```python
from build123d import *

# Parameters (mm, degrees)
BOSS_EXTRUDE1_DEPTH  = 6.5
SKETCH2_R            = 5.5
CUT_EXTRUDE2_DEPTH   = 5
SKETCH3_R            = 4
CUT_EXTRUDE4_DEPTH   = 1.5
M2_CLEARANCE_HOLE1_D = 2.4
M2_CLEARANCE_HOLE2_D = 2.4


with BuildPart() as part:
    # Sketch1 → Boss-Extrude1 (new body)
    with BuildSketch(Plane(origin=(0, 24.8, 0), x_dir=(1, 0, 0), z_dir=(0, 1, 0))):
        with BuildLine():
            Line((5.5, 9), (-22, 9))
            Line((-22, 9), (-22, -9))
            Line((-22, -9), (5.5, -9))
            ThreePointArc((5.5, -9), (14.5, 0), (5.5, 9))
        make_face()
    extrude(amount=BOSS_EXTRUDE1_DEPTH)

    # Sketch2 → Cut-Extrude2 (cut)
    with BuildSketch(Plane(origin=(0, 24.8, 0), x_dir=(1, 0, 0), z_dir=(0, 1, 0))):
        with Locations(Location((5.5, 0, 0), (0, 0, 270))):
            Circle(SKETCH2_R)
    extrude(amount=CUT_EXTRUDE2_DEPTH, mode=Mode.SUBTRACT)

    # Sketch3 → Cut-Extrude4 (cut)
    with BuildSketch(Plane(origin=(0, 29.8, 0), x_dir=(1, 0, 0), z_dir=(0, 1, 0))):
        with Locations(Location((5.5, 0, 0), (0, 0, 270))):
            Circle(SKETCH3_R)
    extrude(amount=CUT_EXTRUDE4_DEPTH, mode=Mode.SUBTRACT)

    # M2 Clearance Hole1 (through all)
    with Locations(Plane(origin=(0, 31.3, 0), x_dir=(1, 0, 0), z_dir=(0, 1, 0))):
        with Locations((-19.5, -4.5)):
            Hole(M2_CLEARANCE_HOLE1_D / 2)

    # M2 Clearance Hole2 (through all)
    with Locations(Plane(origin=(0, 31.3, 0), x_dir=(1, 0, 0), z_dir=(0, 1, 0))):
        with Locations((-19.5, 4.5)):
            Hole(M2_CLEARANCE_HOLE2_D / 2)


solid = part.part
```
Design review of the part built by this model. Coordinates are the model's own, in mm. A direction names the side the tool comes from. Give positions to 0.01 mm unless a question says otherwise; leave off trailing zeros. Write each loop counter-clockwise with the first axis right and the second up, starting at its lowest first coordinate (ties: lowest second). Pieces come first, ordered by that corner, then holes. Notation, with made-up numbers: (-20.5, 51.5) - (14.5, 51.5) arc R18 ccw to (14.5, 62.5) - close; hole circle Ø2 at (31.5, 50). An arc over 180 degrees is marked (long way). Return JSON: item names as keys, results as strings. Group by question number.
(1) Insertion check: pin 1 (1.5 mm diameter, centred on x = 6.5, y = 29, fed in from -Z); pin 2 (5.5 mm diameter, centred on x = 7.5, z = 1, fed in from -Y). Each pin has a flat end and moves straight along its axis. Give the tip position at first contact, or say it passes through.
(2) Mouldability with a two-part tool opening along Z and no side actions: class faces 3 (the cylindrical face through (1.595, 30.54, -0.867)), 4 (the flat face through (-4, 31.3, 0)), 5 (the flat face through (-8, 28, -9)), 6 (the cylindrical face through (14.498, 28.004, 0.198)) as +Z half, -Z half, draft (parallel to the pull), parting line (faces both ways), or undercut.
(3) We need section B-B, the plane z = 0. Give the boundary of the cut face in (x, y).
(4) To check wall thickness, follow probe 1 along Z at (x, y) = (-19.5, 27.25); probe 2 along X at (y, z) = (26.9, 0); probe 3 along Z at (x, y) = (10, 26.5). State the ranges of each line that lie inside material, in increasing order.
(5) We need section C-C, the plane x = 4.5. Give the boundary of the cut face in (y, z).
(6) We need section A-A, the plane y = 30.25. Give the boundary of the cut face in (x, z), then the cut area to 3 significant figures.
(7) Machinability: for faces 1 (the cylindrical face through (-18.3, 28, 4.45)), 2 (the flat face through (1, 29.8, 0)), which of the approach directions +Z, -Z, +X, -X, +Y, -Y give a long, thin tool a straight path to every point of the face, cutting with its end or side? Answer none if there is none.
(8) We need section D-D, the plane y = 28.5. Give the boundary of the cut face in (x, z), then the cut area to 3 significant figures.
Reported:
{
 "1": {"pin 1": "stops at z = -9", "pin 2": "stops at y = 29.8"},
 "2": {"face 3": "undercut", "face 4": "draft", "face 5": "-Z half", "face 6": "parting line"},
 "3": {"outline": "(-22, 24.8) - (0, 24.8) - (0, 29.8) - (1.5, 29.8) - (1.5, 31.3) - (-22, 31.3) - close; (9.5, 29.8) - (11, 29.8) - (11, 24.8) - (14.5, 24.8) - (14.5, 31.3) - (9.5, 31.3) - close"},
 "4": {"probe 1": "z = -9 to -5.7, -3.3 to 3.3, 5.7 to 9", "probe 2": "x = -22 to 0, 11 to 14.5", "probe 3": "z = -7.79 to -3.16, 3.16 to 7.79"},
 "5": {"outline": "(24.8, -9) - (31.3, -9) - (31.3, -3.87) - (29.8, -3.87) - (29.8, -5.41) - (24.8, -5.41) - close; (24.8, 5.41) - (29.8, 5.41) - (29.8, 3.87) - (31.3, 3.87) - (31.3, 9) - (24.8, 9) - close"},
 "6": {"outline": "(-22, -9) - (5.5, -9) arc R9 ccw to (5.5, 9) - (-22, 9) - close; hole circle Ø2.4 at (-19.5, -4.5); hole circle Ø2.4 at (-19.5, 4.5); hole circle Ø8 at (5.5, 0)", "area": "563 mm2"},
 "7": {"face 1": "+Y, -Y", "face 2": "-Y"},
 "8": {"outline": "(-22, -9) - (5.5, -9) arc R9 ccw to (5.5, 9) - (-22, 9) - close; hole circle Ø2.4 at (-19.5, -4.5); hole circle Ø2.4 at (-19.5, 4.5); hole circle Ø11 at (5.5, 0)", "area": "518 mm2"}
}
